Check sheet for the modelled part. Datum: model origin and axes. Units: mm. A direction names the side the tool comes from. Round coordinates to 2 decimals unless told otherwise and drop trailing zeros. Write each loop counter-clockwise with the first axis right and the second up, starting at its lowest first coordinate (ties: lowest second). Pieces come first, ordered by that corner, then holes.
Item 1: Release check for a two-part mould opening along X. For faces 6 (the flat face through (8, 57, 2)), 7 (the flat face through (6.9, 13, 2)), 8 (the flat face through (7, 53.799, 2)) record: +X half, -X half, draft (parallel to the pull), parting line (faces both ways), or undercut.
Item 2: Cross-section at C-C on y = 33. Enter the section's corners in (x, z), plus the area to 3 significant figures.
Item 3: Cross-section at B-B on x = 11.25. Enter the section's corners in (y, z), plus the area to 3 significant figures.
Item 4: Cross-section at A-A on z = 4.2. Enter the section's corners in (x, y), plus the area to 3 significant figures.
Item 5: Material ranges on line 1 (Y direction, x = 3.5, z = 2.9); line 2 (Y direction, x = 4, z = 2.95); line 3 (X direction, y = 11, z = 3.35), recorded low to high.
Item 6: Go/stop test with flat-tipped pins: pin 1 Ø2.5 at (x, z) = (17, 2.5) entering from +Y; pin 2 Ø2.5 at (y, z) = (55, 3.5) entering from -X; pin 3 Ø0.9 at (x, z) = (6.5, 3.5) entering from -Y; pin 4 Ø1.5 at (y, z) = (6, 3.5) entering from +X. Record where each tip stops, or that it passes through.
Item 7: Tool access check on faces 1 (the flat face through (4, 15.299, 2)), 2 (the flat face through (4, 59.799, 2)), 3 (the flat face through (6, 11.299, 2)), 4 (the flat face through (26.9, 15, 2)), 5 (the flat face through (19, 15.299, 2)). Record the directions out of +Z, -Z, +X, -X, +Y, -Y that give a thin tool (end or side, any length) a straight path to the whole face; none if there is none.
Item 8: Cross-section at D-D on x = 16.25. Enter the section's corners in (y, z).
from build123d import *

# Parameters (mm, degrees)
EXTRUDE_1_DEPTH     = 5
CUT_EXTRUDE_1_DEPTH = 66.760863021


with BuildPart() as part:
    # 草图1 → 凸台-拉伸1 (new body)
    with BuildSketch(Plane.XY):
        Polygon((0, 0), (0, 59.798671434), (8, 59.798671434), (8, 53.798671434), (5, 53.798671434), (5, 56.798671434), (3, 56.798671434), (3, 15.298671434), (5, 15.298671434), (5, 11.298671434), (6.9, 11.298671434), (6.9, 13.798671434), (11.9, 15.298671434), (26.9, 15.298671434), (26.9, 13.798671434), (3, 0), align=None)
    extrude(amount=EXTRUDE_1_DEPTH)

    # 草图2 → 切除-拉伸1 (cut, through all)
    with BuildSketch(Plane.XY.offset(5)):
        Polygon((22.033974596, 13.298671434), (12.193537673, 13.298671434), (8.9, 12.310610132), (8.9, 9.298671434), (3, 9.298671434), (3, 13.298671434), (2, 13.298671434), (2, 2), (2.464101615, 2), align=None)
    extrude(amount=-CUT_EXTRUDE_1_DEPTH, mode=Mode.SUBTRACT)


solid = part.part
Response values:
1. face 6: +X half
1. face 7: undercut
1. face 8: draft
2. outline: (0, 0) - (3, 0) - (3, 5) - (0, 5) - close
2. area: 15.0 mm2
3. outline: (4.76, 0) - (7.07, 0) - (7.07, 5) - (4.76, 5) - close; (13.02, 0) - (15.1, 0) - (15.1, 5) - (13.02, 5) - close
3. area: 22.0 mm2
4. outline: (0, 0) - (3, 0) - (26.9, 13.8) - (26.9, 15.3) - (11.9, 15.3) - (6.9, 13.8) - (6.9, 11.3) - (5, 11.3) - (5, 15.3) - (3, 15.3) - (3, 56.8) - (5, 56.8) - (5, 53.8) - (8, 53.8) - (8, 59.8) - (0, 59.8) - close; hole (2, 2) - (2.46, 2) - (22.03, 13.3) - (12.19, 13.3) - (8.9, 12.31) - (8.9, 9.3) - (3, 9.3) - (3, 13.3) - (2, 13.3) - close
4. area: 302 mm2
5. line 1: y = 0.29 to 2.6, 9.3 to 15.3, 56.8 to 59.8
5. line 2: y = 0.58 to 2.89, 9.3 to 15.3, 56.8 to 59.8
5. line 3: x = 0 to 2, 3 to 8.9, 18.05 to 22.05
6. pin 1: stops at y = 15.3
6. pin 2: stops at x = 0
6. pin 3: stops at y = 1.76
6. pin 4: stops at x = 14.69
7. face 1: +Z, -Z, +X
7. face 2: +Z, -Z, +X, -X, +Y
7. face 3: +Z, -Z
7. face 4: +Z, -Z, +X, +Y, -Y
7. face 5: +Z, -Z, +X, +Y
8. outline: (7.65, 0) - (9.96, 0) - (9.96, 5) - (7.65, 5) - close; (13.3, 0) - (15.3, 0) - (15.3, 5) - (13.3, 5) - close
